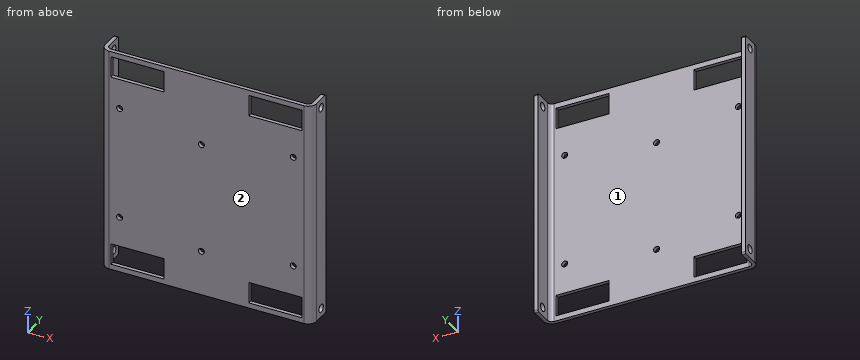
```python
from build123d import *

# Parameters (mm, degrees)
F1_DEPTH  = 101.6
F2_R      = 3.69316
F3_R      = 1.98374
F4_W      = 24
F4_H      = 9.5329248
F4_R      = 1.35255
F5_DEPTH  = 1.70942
F6_R      = 1.8288
F7_DEPTH  = 95.37192
F8_R      = 0.762
F9_R      = 1.35255
F10_DEPTH = 1.70942


with BuildPart() as f1:
    # F0 (on Top) → F1 (new body)
    with BuildSketch(Plane.XY):
        Polygon((0, 9.92124), (0, 0), (-91.95308, 0), (-91.95308, 9.92124), (-93.6625, 9.92124), (-93.6625, -1.70942), (1.70942, -1.70942), (1.70942, 9.92124), align=None)
    extrude(amount=F1_DEPTH)

    # F2
    f2_edges = [f1.edges().sort_by_distance(p)[0] for p in [
        (1.70942, -1.70942, 50.8),
        (-93.6625, -1.70942, 50.8),
    ]]
    fillet(f2_edges, radius=F2_R)

    # F3
    f3_edges = [f1.edges().sort_by_distance(p)[0] for p in [
        (0, 0, 50.8),
        (-91.95308, 0, 50.8),
    ]]
    fillet(f3_edges, radius=F3_R)

    # F4 (on face) → F5 (cut, through all)
    with BuildSketch(Plane(origin=(0, 0, 0), x_dir=(-1, 0, 0), z_dir=(0, 1, 0))):
        with Locations((77.17559, 94.4522876)):
            Rectangle(F4_W, F4_H)
        with Locations((77.17559, 7.1477124)):
            Rectangle(F4_W, F4_H)
        with Locations((14.77749, 7.1477124)):
            Rectangle(F4_W, F4_H)
        with Locations((14.77749, 94.4522876)):
            Rectangle(F4_W, F4_H)
        with Locations((85.20684, 76.1477196107)):
            Circle(F4_R)
        with Locations((85.20684, 25.4522803893)):
            Circle(F4_R)
        with Locations((6.74624, 25.4522803893)):
            Circle(F4_R)
        with Locations((6.74624, 76.1477196107)):
            Circle(F4_R)
    extrude(amount=-F5_DEPTH, mode=Mode.SUBTRACT)

    # F6 (on face) → F7 (cut, through all)
    with BuildSketch(Plane.YZ.offset(1.70942)):
        with Locations((5.95249, 97.63125)):
            Circle(F6_R)
        with Locations((5.95249, 3.96875)):
            Circle(F6_R)
    extrude(amount=-F7_DEPTH, mode=Mode.SUBTRACT)

    # F8
    f8_edges = [f1.edges().sort_by_distance(p)[0] for p in [
        (-92.80779, 9.92124, 101.6),
        (-92.80779, 9.92124, 0),
        (0.85471, 9.92124, 0),
        (0.85471, 9.92124, 101.6),
    ]]
    fillet(f8_edges, radius=F8_R)

    # F9 (on face) → F10 (cut, through all)
    with BuildSketch(Plane(origin=(0, 0, 0), x_dir=(-1, 0, 0), z_dir=(0, 1, 0))):
        with Locations((48.26635, 70.0399442418)):
            Circle(F9_R)
        with Locations((48.26635, 20.2559442418)):
            Circle(F9_R)
    extrude(amount=-F10_DEPTH, mode=Mode.SUBTRACT)


solid = f1.part
```
Check sheet for the modelled part. Datum: model origin and axes. Units: mm. Face numbers are marked on the shaded views. Give positions to 0.01 mm unless a question says otherwise; leave off trailing zeros. Write each loop counter-clockwise with the first axis right and the second up, starting at its lowest first coordinate (ties: lowest second). Pieces come first, ordered by that corner, then holes.
Item 1: Cross-section at D-D (x = -35). Enter the section's corners in (y, z).
Item 2: Scan lines: L1, parallel to Z at x = -12, y = -0.5; L2, parallel to X at y = 5.25, z = 51.5; L3, parallel to Y at x = -5.5, z = 52.5. Record each from-to range of solid material in increasing order.
Item 3: Cross-section at B-B (z = 62). Enter the section's corners in (x, y), and give its area (3 significant figures).
Item 4: Cross-section at A-A (x = -79). Enter the section's corners in (y, z), and give its area (3 significant figures).
Item 5: Cross-section at C-C (y = 6). Enter the section's corners in (x, z).
Item 6: Draft check along X on the marked faces 1 and 2. Enter one of: released by +X, released by -X, zero draft, split by the parting line, or undercut.
Item 7: Gauge pin test, flat ends, axial feed: pin 1 (1.4 mm diameter, centred on y = -1, z = 8, fed in from +X); pin 2 (2 mm diameter, centred on y = 0.5, z = 44, fed in from +X); pin 3 (0.5 mm diameter, centred on y = -1, z = 96.5, fed in from -X). Record the tip position at first contact, or that the pin passes through.
Report:
1. outline: (-1.71, 0) - (0, 0) - (0, 101.6) - (-1.71, 101.6) - close
2. L1: z = 0 to 2.38, 11.91 to 89.69, 99.22 to 101.6
2. L2: x = -93.66 to -91.95, 0 to 1.71
2. L3: y = -1.71 to 0
3. outline: (-93.66, 1.98) arc R3.69 ccw to (-89.97, -1.71) - (-1.98, -1.71) arc R3.69 ccw to (1.71, 1.98) - (1.71, 9.92) - (0, 9.92) - (0, 1.98) arc R1.98 cw to (-1.98, 0) - (-89.97, 0) arc R1.98 cw to (-91.95, 1.98) - (-91.95, 9.92) - (-93.66, 9.92) - close
3. area: 193 mm2
4. outline: (-1.71, 0) - (0, 0) - (0, 2.38) - (-1.71, 2.38) - close; (-1.71, 11.91) - (0, 11.91) - (0, 89.69) - (-1.71, 89.69) - close; (-1.71, 99.22) - (0, 99.22) - (0, 101.6) - (-1.71, 101.6) - close
4. area: 141 mm2
5. outline: (-93.66, 0) - (-91.95, 0) - (-91.95, 2.14) - (-93.66, 2.14) - close; (-93.66, 5.8) - (-91.95, 5.8) - (-91.95, 95.8) - (-93.66, 95.8) - close; (-93.66, 99.46) - (-91.95, 99.46) - (-91.95, 101.6) - (-93.66, 101.6) - close; (0, 0) - (1.71, 0) - (1.71, 2.14) - (0, 2.14) - close; (0, 5.8) - (1.71, 5.8) - (1.71, 95.8) - (0, 95.8) - close; (0, 99.46) - (1.71, 99.46) - (1.71, 101.6) - (0, 101.6) - close
6. face 1: undercut
6. face 2: zero draft
7. pin 1: stops at x = 0.92
7. pin 2: stops at x = 1.68
7. pin 3: stops at x = -92.45
